Source: CAD feature listing. Evaluate the final solid. Frame: model axes, mm. Face numbers are marked on the shaded views. A direction names the side the tool comes from. Round coordinates to 2 decimals unless told otherwise and drop trailing zeros. Order: outer loops, then holes, each group sorted by start corner. A loop starts at its lowest first (then second) coordinate and runs counter-clockwise, first axis right, second up. Notation, with made-up numbers: (59.25, 28.25) -> (68.25, 28.25) arc R14 cw to (68.25, 49.25) -> close; hole circle Ø4 at (67.25, 50). An arc over 180 degrees is marked (long way). Write item = value, one per line. Start each with the question number.
(1) Draft query along Z for the marked faces 1, 2 and 3. Return one class per face: released by +Z, released by -Z, zero draft, split by the parting line, or undercut.
(2) Cut plane A-A on x = -34.5. Return the cut outline in (y, z), then the cut area to 3 significant figures.
(3) Contact query for flat-ended pins moving along their axis: pin 1 Ø10.5 at (x, y) = (13, 12) entering from +Z; pin 2 Ø14.5 at (x, z) = (40, 27.5) entering from +Y. Output: stop coordinate, or through.
(4) Cut plane C-C on x = 0. Return the cut outline in (y, z), then the cut area to 3 significant figures.
(5) Reachability of the marked faces 4 and 5 from +Z, -Z, +X, -X, +Y, -Y: full face, straight path, thin tool, end or side. Return the list, or none.
(6) Cut plane B-B on z = 2. Return the cut outline in (x, y).
(7) Cut plane D-D on x = 29.5. Return the cut outline in (y, z), then the cut area to 3 significant figures.
(8) Ray query, line 1 (Z direction, x = 0, y = 1.6); line 2 (Z direction, x = 10.5, y = 9); line 3 (X direction, y = 11.25, z = -24). Return the intervals inside material, ascending.
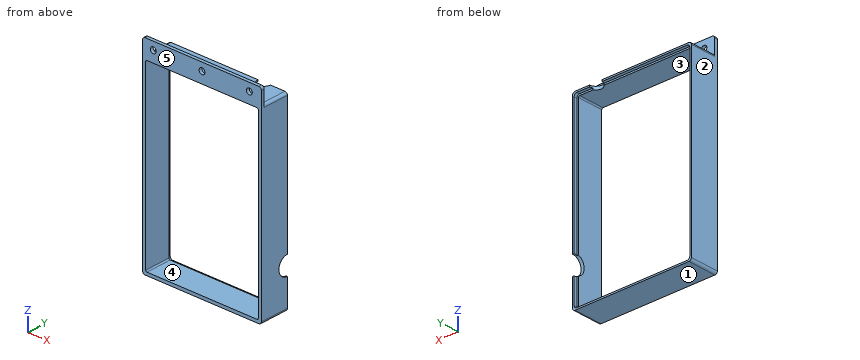
from build123d import *

# Parameters (mm, degrees)
SKETCH1_W                          = 97.571055574
SKETCH1_H                          = 151.345533826
SKETCH1_W_2                        = 92.491055574
SKETCH1_H_2                        = 146.265533826
BOSS_EXTRUDE1_DEPTH                = 23.619000006
SKETCH2_W                          = 97.571055574
SKETCH2_H                          = 12.724538291
BOSS_EXTRUDE2_DEPTH                = 2.54
FILLET1_R                          = 2
FILLET2_R                          = 1
F_3_16_0_1875_DIAMETER_HOLE1_D     = 4.7625
F_3_16_0_1875_DIAMETER_HOLE1_DEPTH = 20.066
F_3_16_0_1875_DIAMETER_HOLE1_TIP   = 1.430799349
CUT_EXTRUDE1_DEPTH                 = 2.54
CUT_EXTRUDE2_REACH                 = 99.571
SKETCH8_R                          = 7.6835
CUT_EXTRUDE3_REACH                 = 153.346
SKETCH9_R                          = 5.08


with BuildPart() as part:
    # Sketch1 → Boss-Extrude1 (new body)
    with BuildSketch(Plane(origin=(0, 0, 0), x_dir=(1, 0, 0), z_dir=(0, 1, 0))):
        Rectangle(SKETCH1_W, SKETCH1_H)
        Rectangle(SKETCH1_W_2, SKETCH1_H_2, mode=Mode.SUBTRACT)
    extrude(amount=BOSS_EXTRUDE1_DEPTH)

    # Sketch2 → Boss-Extrude2 (add)
    with BuildSketch(Plane.XZ):
        with Locations((0, 82.035036058)):
            Rectangle(SKETCH2_W, SKETCH2_H)
    extrude(amount=-BOSS_EXTRUDE2_DEPTH)

    # Fillet1
    fillet1_edges = [part.edges().sort_by_distance(p)[0] for p in [
        (-48.785527787, 1.27, 88.397305204),
        (48.785527787, 1.27, 88.397305204),
        (48.785527787, 13.079500003, 75.672766913),
        (-48.785527787, 13.079500003, 75.672766913),
        (-48.785527787, 11.809500003, -75.672766913),
        (48.785527787, 11.809500003, -75.672766913),
    ]]
    fillet(fillet1_edges, radius=FILLET1_R)

    # Fillet2
    fillet2_edges = [part.edges().sort_by_distance(p)[0] for p in [
        (46.245527787, 11.809500003, 73.132766913),
        (46.245527787, 11.809500003, -73.132766913),
        (-46.245527787, 11.809500003, -73.132766913),
        (-46.245527787, 11.809500003, 73.132766913),
    ]]
    fillet(fillet2_edges, radius=FILLET2_R)

    # 3/16 (0.1875) Diameter Hole1
    with Locations(Plane(origin=(0, 2.54, 0), x_dir=(1, 0, 0), z_dir=(0, 1, 0))):
        with Locations((-40.04587174, -82.10120048), (38.957668704, -82.10120048), (0, -82.10120048)):
            Hole(F_3_16_0_1875_DIAMETER_HOLE1_D / 2, depth=F_3_16_0_1875_DIAMETER_HOLE1_DEPTH)
            with Locations((0, 0, -(F_3_16_0_1875_DIAMETER_HOLE1_DEPTH + F_3_16_0_1875_DIAMETER_HOLE1_TIP / 2))):  # 118° drill point
                Cone(0, F_3_16_0_1875_DIAMETER_HOLE1_D / 2, F_3_16_0_1875_DIAMETER_HOLE1_TIP, mode=Mode.SUBTRACT)

    # Sketch5 → Cut-Extrude1 (cut)
    with BuildSketch(Plane(origin=(0, 23.619000006, 0), x_dir=(1, 0, 0), z_dir=(0, 1, 0))):
        with BuildLine():
            Line((-45.245527787, -74.402766913), (45.245527787, -74.402766913))
            ThreePointArc((45.245527787, -74.402766913), (46.85066018, -73.737899306), (47.515527787, -72.132766913))
            Line((47.515527787, -72.132766913), (47.515527787, 72.132766913))
            ThreePointArc((47.515527787, 72.132766913), (46.85066018, 73.737899306), (45.245527787, 74.402766913))
            Line((45.245527787, 74.402766913), (-45.245527787, 74.402766913))
            ThreePointArc((-45.245527787, 74.402766913), (-46.85066018, 73.737899306), (-47.515527787, 72.132766913))
            Line((-47.515527787, 72.132766913), (-47.515527787, -72.132766913))
            ThreePointArc((-47.515527787, -72.132766913), (-46.85066018, -73.737899306), (-45.245527787, -74.402766913))
        make_face()
        with BuildLine():
            Line((-46.245527787, 72.132766913), (-46.245527787, -72.132766913))
            ThreePointArc((-46.245527787, -72.132766913), (-45.952634568, -72.839873694), (-45.245527787, -73.132766913))
            Line((-45.245527787, -73.132766913), (45.245527787, -73.132766913))
            ThreePointArc((45.245527787, -73.132766913), (45.952634568, -72.839873694), (46.245527787, -72.132766913))
            Line((46.245527787, -72.132766913), (46.245527787, 72.132766913))
            ThreePointArc((46.245527787, 72.132766913), (45.952634568, 72.839873694), (45.245527787, 73.132766913))
            Line((45.245527787, 73.132766913), (-45.245527787, 73.132766913))
            ThreePointArc((-45.245527787, 73.132766913), (-45.952634568, 72.839873694), (-46.245527787, 72.132766913))
        make_face(mode=Mode.SUBTRACT)
    extrude(amount=-CUT_EXTRUDE1_DEPTH, mode=Mode.SUBTRACT)

    # Sketch8 → Cut-Extrude2 (cut, up to next)
    with BuildSketch(Plane(origin=(48.785527787, 0, 0), x_dir=(0, 0, -1), z_dir=(1, 0, 0)), mode=Mode.PRIVATE) as cut_extrude2_sk1:
        with Locations((43.922766913, 23.619000006)):
            Circle(SKETCH8_R)
    cut_extrude2_tool1 = extrude(cut_extrude2_sk1.sketch, amount=-CUT_EXTRUDE2_REACH, mode=Mode.PRIVATE) & part.part
    add(cut_extrude2_tool1.solids().sort_by_distance((48.785528, 23.619, -43.922767))[0], mode=Mode.SUBTRACT)

    # Sketch9 → Cut-Extrude3 (cut, up to next)
    with BuildSketch(Plane.XY.offset(75.672766913), mode=Mode.PRIVATE) as cut_extrude3_sk1:
        with Locations((29.735527787, 23.619000006)):
            Circle(SKETCH9_R)
    cut_extrude3_tool1 = extrude(cut_extrude3_sk1.sketch, amount=-CUT_EXTRUDE3_REACH, mode=Mode.PRIVATE) & part.part
    add(cut_extrude3_tool1.solids().sort_by_distance((29.735528, 23.619, 75.672767))[0], mode=Mode.SUBTRACT)


solid = part.part
Evaluation:
q1.face_1 = released by -Z
q1.face_2 = zero draft
q1.face_3 = undercut
q2.outline = (0, -75.67) -> (23.62, -75.67) -> (23.62, -74.4) -> (21.08, -74.4) -> (21.08, -73.13) -> (0, -73.13) -> close; (0, 73.13) -> (21.08, 73.13) -> (21.08, 74.4) -> (23.62, 74.4) -> (23.62, 75.67) -> (2.54, 75.67) -> (2.54, 88.4) -> (0, 88.4) -> close
q2.area = 146 mm^2
q3.pin_1 = 75.67
q3.pin_2 = 21.08
q4.outline = (0, -75.67) -> (23.62, -75.67) -> (23.62, -74.4) -> (21.08, -74.4) -> (21.08, -73.13) -> (0, -73.13) -> close; (0, 73.13) -> (21.08, 73.13) -> (21.08, 74.4) -> (23.62, 74.4) -> (23.62, 75.67) -> (2.54, 75.67) -> (2.54, 79.72) -> (0, 79.72) -> close; (0, 84.48) -> (2.54, 84.48) -> (2.54, 88.4) -> (0, 88.4) -> close
q4.area = 134 mm^2
q5.face_4 = +Y, -Y
q5.face_5 = +Z, -Z, +X, -X, -Y
q6.outline = (-48.79, 0) -> (-46.25, 0) -> (-46.25, 21.08) -> (-47.52, 21.08) -> (-47.52, 23.62) -> (-48.79, 23.62) -> close; (46.25, 0) -> (48.79, 0) -> (48.79, 23.62) -> (47.52, 23.62) -> (47.52, 21.08) -> (46.25, 21.08) -> close
q7.outline = (0, -75.67) -> (23.62, -75.67) -> (23.62, -74.4) -> (21.08, -74.4) -> (21.08, -73.13) -> (0, -73.13) -> close; (0, 73.13) -> (18.54, 73.13) -> (18.54, 75.67) -> (2.54, 75.67) -> (2.54, 88.4) -> (0, 88.4) -> close
q7.area = 136 mm^2
q8.line_1 = -75.67 to -73.13, 73.13 to 79.72, 84.48 to 88.4
q8.line_2 = -75.67 to -73.13, 73.13 to 75.67
q8.line_3 = -48.79 to -46.25, 46.25 to 48.79
